Here's the drawing with two shaded views (mm, measured from the low corner). I have some questions. Give positions to 0.01 mm unless a question says otherwise; leave off trailing zeros. Loops run counter-clockwise (first coordinate to the right, second up) from the corner with the lowest first, then second, coordinate; pieces in that order, holes last. Notation, with made-up numbers: (-11, 68.5) -> (18, 68.5) arc R20 cw to (18, 85.5) -> close; hole circle Ø1 at (28.5, 65). An arc over 180 degrees is marked (long way). Answer in a Markdown table with one row per item. Add a question column.
Item 1: If I drill on line 1 (X direction, y = 101, z = 1); line 2 (X direction, y = 49.5, z = 1.75); line 3 (Y direction, x = 7, z = 1), over which ranges is the centre line in solid material (lowest first)?
Item 2: If we section it at B-B (z = 1.15): Write out the boundary of the cut face in (x, y).
Item 3: If we section it at D-D (y = 15): Write out the boundary of the cut face in (x, z), then the cut area to 3 significant figures.
Item 4: If we section it at A-A (y = 49): Write out the boundary of the cut face in (x, z).
Item 5: For P1, Ø2.5, axis at x = 7, y = 101, coming from the -Z side, with a flat end and sliding along its axis, tell me the tip position at first contact or that it passes through.
Item 6: If we section it at C-C (x = 73.3): Write out the boundary of the cut face in (y, z), then the cut area to 3 significant figures.
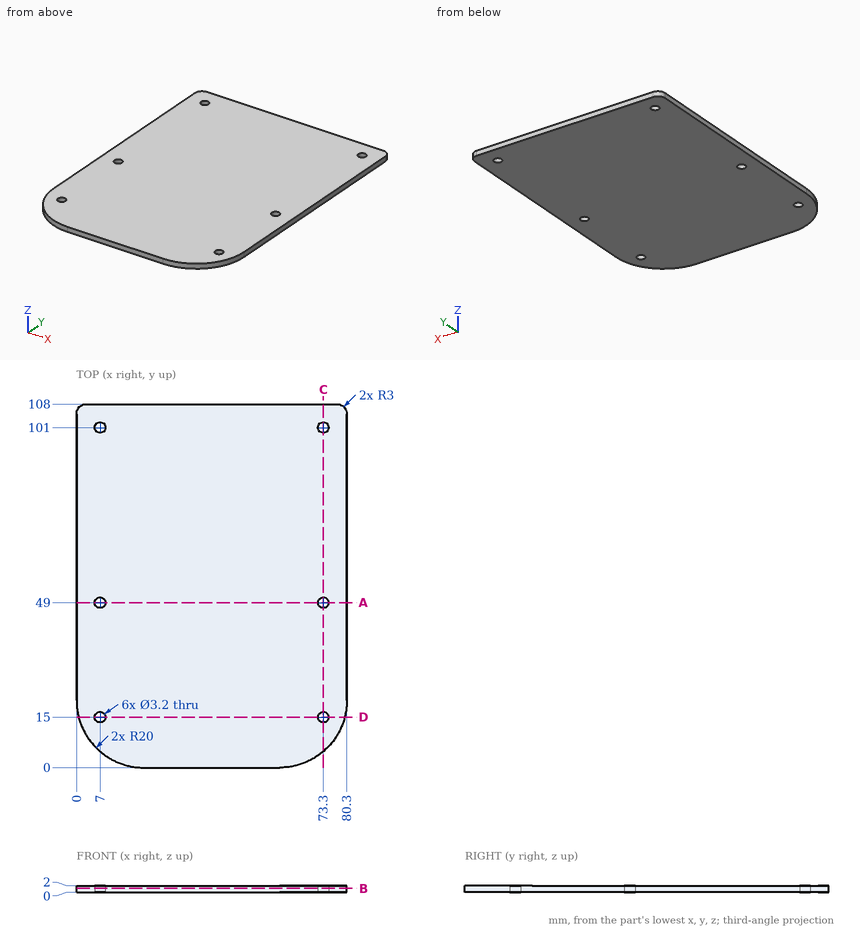
Recorded:
| question | item | result |
|---|---|---|
| 1 | line 1 | x = 0 to 5.4, 8.6 to 71.7, 74.9 to 80.3 |
| 1 | line 2 | x = 0 to 5.48, 8.52 to 71.78, 74.82 to 80.3 |
| 1 | line 3 | y = 4.8 to 13.4, 16.6 to 47.4, 50.6 to 99.4, 102.6 to 108 |
| 2 | outline | (0, 20) arc R20 ccw to (20, 0) -> (60.3, 0) arc R20 ccw to (80.3, 20) -> (80.3, 105) arc R3 ccw to (77.3, 108) -> (3, 108) arc R3 ccw to (0, 105) -> close; hole circle Ø3.2 at (7, 15); hole circle Ø3.2 at (7, 49); hole circle Ø3.2 at (7, 101); hole circle Ø3.2 at (73.3, 15); hole circle Ø3.2 at (73.3, 49); hole circle Ø3.2 at (73.3, 101) |
| 3 | outline | (0.64, 0) -> (5.4, 0) -> (5.4, 2) -> (0.64, 2) -> close; (8.6, 0) -> (71.7, 0) -> (71.7, 2) -> (8.6, 2) -> close; (74.9, 0) -> (79.66, 0) -> (79.66, 2) -> (74.9, 2) -> close |
| 3 | area | 145 mm^2 |
| 4 | outline | (0, 0) -> (5.4, 0) -> (5.4, 2) -> (0, 2) -> close; (8.6, 0) -> (71.7, 0) -> (71.7, 2) -> (8.6, 2) -> close; (74.9, 0) -> (80.3, 0) -> (80.3, 2) -> (74.9, 2) -> close |
| 5 | P1 | passes through |
| 6 | outline | (4.8, 0) -> (13.4, 0) -> (13.4, 2) -> (4.8, 2) -> close; (16.6, 0) -> (47.4, 0) -> (47.4, 2) -> (16.6, 2) -> close; (50.6, 0) -> (99.4, 0) -> (99.4, 2) -> (50.6, 2) -> close; (102.6, 0) -> (108, 0) -> (108, 2) -> (102.6, 2) -> close |
| 6 | area | 187 mm^2 |
